```python
from build123d import *

# Parameters (mm, degrees)
SKETCH1_R           = 2.5
BOSS_EXTRUDE1_DEPTH = 2.5
BOSS_EXTRUDE2_START = -45
SKETCH4_R           = 3.5
SKETCH4_R_2         = 2
BOSS_EXTRUDE2_DEPTH = 47.5
BOSS_EXTRUDE3_START = -2.5
SKETCH5_R           = 2.5
BOSS_EXTRUDE3_DEPTH = 2.5
BOSS_EXTRUDE4_START = -12
BOSS_EXTRUDE4_DEPTH = 12
BOSS_EXTRUDE5_DEPTH = 2.5
FILLET2_R           = 1
FILLET3_R           = 1


with BuildPart() as part:
    # Sketch1 → Boss-Extrude1 (new body)
    with BuildSketch(Plane(origin=(0, 0, 0), x_dir=(1, 0, 0), z_dir=(0, 1, 0))):
        with BuildLine():
            Line((20.5, 10.5), (-20.5, 10.5))
            Line((-20.5, 10.5), (-20.5, 4))
            ThreePointArc((-20.5, 4), (-24.40287122, 1.76806345), (-28.520566145, 3.573204173))
            ThreePointArc((-28.520566145, 3.573204173), (-29.324072849, 5.171652721), (-29.350396575, 6.960498116))
            ThreePointArc((-29.350396575, 6.960498116), (-26.904940816, 10.941842627), (-22.5, 12.5))
            Line((-22.5, 12.5), (22.5, 12.5))
            ThreePointArc((22.5, 12.5), (26.904940816, 10.941842627), (29.350396575, 6.960498116))
            ThreePointArc((29.350396575, 6.960498116), (29.324072849, 5.171652721), (28.520566145, 3.573204173))
            ThreePointArc((28.520566145, 3.573204173), (25.737402548, 1.876578025), (22.5, 2.2557411))
            Line((22.5, 2.2557411), (22.5, -2.2557411))
            ThreePointArc((22.5, -2.2557411), (25.737402548, -1.876578025), (28.520566145, -3.573204173))
            ThreePointArc((28.520566145, -3.573204173), (29.324072849, -5.171652721), (29.350396575, -6.960498116))
            ThreePointArc((29.350396575, -6.960498116), (26.904940816, -10.941842627), (22.5, -12.5))
            Line((22.5, -12.5), (-22.5, -12.5))
            ThreePointArc((-22.5, -12.5), (-26.904940816, -10.941842627), (-29.350396575, -6.960498116))
            ThreePointArc((-29.350396575, -6.960498116), (-29.324072849, -5.171652721), (-28.520566145, -3.573204173))
            ThreePointArc((-28.520566145, -3.573204173), (-24.40287122, -1.76806345), (-20.5, -4))
            Line((-20.5, -4), (-20.5, -10.5))
            Line((-20.5, -10.5), (20.5, -10.5))
            Line((20.5, -10.5), (20.5, 10.5))
        make_face()
        with Locations(Location((-25, 5.5, 0), (0, 0, 270))):
            Circle(SKETCH1_R, mode=Mode.SUBTRACT)
        with Locations(Location((-25, -5.5, 0), (0, 0, 270))):
            Circle(SKETCH1_R, mode=Mode.SUBTRACT)
        with Locations(Location((25, -5.5, 0), (0, 0, 90))):
            Circle(SKETCH1_R, mode=Mode.SUBTRACT)
        with Locations(Location((25, 5.5, 0), (0, 0, 90))):
            Circle(SKETCH1_R, mode=Mode.SUBTRACT)
    extrude(amount=BOSS_EXTRUDE1_DEPTH)

    # Sketch4 → Boss-Extrude2 (add)
    # profile 1 of 4: a face of its own
    with BuildSketch(Plane(origin=(0, 0, 0), x_dir=(1, 0, 0), z_dir=(0, 1, 0)).offset(BOSS_EXTRUDE2_START)):
        with Locations(Location((-20.5, 15.5, 0), (0, 0, 270))):
            Circle(SKETCH4_R)
        with Locations(Location((-20.5, 15.5, 0), (0, 0, 270))):
            Circle(SKETCH4_R_2, mode=Mode.SUBTRACT)
    # profile 2 of 4: a face of its own
    with BuildSketch(Plane(origin=(0, 0, 0), x_dir=(1, 0, 0), z_dir=(0, 1, 0)).offset(BOSS_EXTRUDE2_START)):
        with Locations(Location((20.5, 15.5, 0), (0, 0, 270))):
            Circle(SKETCH4_R)
        with Locations(Location((20.5, 15.5, 0), (0, 0, 270))):
            Circle(SKETCH4_R_2, mode=Mode.SUBTRACT)
    # profile 3 of 4: a face of its own
    with BuildSketch(Plane(origin=(0, 0, 0), x_dir=(1, 0, 0), z_dir=(0, 1, 0)).offset(BOSS_EXTRUDE2_START)):
        with Locations(Location((-20.5, -15.5, 0), (0, 0, 270))):
            Circle(SKETCH4_R)
        with Locations(Location((-20.5, -15.5, 0), (0, 0, 270))):
            Circle(SKETCH4_R_2, mode=Mode.SUBTRACT)
    # profile 4 of 4: a face of its own
    with BuildSketch(Plane(origin=(0, 0, 0), x_dir=(1, 0, 0), z_dir=(0, 1, 0)).offset(BOSS_EXTRUDE2_START)):
        with Locations(Location((20.5, -15.5, 0), (0, 0, 270))):
            Circle(SKETCH4_R)
        with Locations(Location((20.5, -15.5, 0), (0, 0, 270))):
            Circle(SKETCH4_R_2, mode=Mode.SUBTRACT)
    extrude(amount=BOSS_EXTRUDE2_DEPTH)

    # Sketch5 → Boss-Extrude3 (add)
    with BuildSketch(Plane(origin=(0, 0, 0), x_dir=(1, 0, 0), z_dir=(0, 1, 0)).offset(BOSS_EXTRUDE3_START)):
        with BuildLine():
            Line((-29.324072849, 5.171652721), (-29.324072849, -5.171652721))
            ThreePointArc((-29.324072849, -5.171652721), (-29.438527194, -6.064584851), (-29.350396575, -6.960498116))
            ThreePointArc((-29.350396575, -6.960498116), (-27.465923203, -10.435821373), (-24, -12.337527971))
            Line((-24, -12.337527971), (-24, -15.5))
            Line((-24, -15.5), (-22.5, -15.5))
            ThreePointArc((-22.5, -15.5), (-20.5, -13.5), (-18.5, -15.5))
            Line((-18.5, -15.5), (-17, -15.5))
            Line((-17, -15.5), (-17, -12.5))
            Line((-17, -12.5), (17, -12.5))
            Line((17, -12.5), (17, -15.5))
            Line((17, -15.5), (18.5, -15.5))
            ThreePointArc((18.5, -15.5), (20.5, -13.5), (22.5, -15.5))
            Line((22.5, -15.5), (24, -15.5))
            Line((24, -15.5), (24, -12.337527971))
            ThreePointArc((24, -12.337527971), (27.465923203, -10.435821373), (29.350396575, -6.960498116))
            ThreePointArc((29.350396575, -6.960498116), (29.324072849, -5.171652721), (28.520566145, -3.573204173))
            ThreePointArc((28.520566145, -3.573204173), (25.737402548, -1.876578025), (22.5, -2.2557411))
            Line((22.5, -2.2557411), (22.5, 2.2557411))
            ThreePointArc((22.5, 2.2557411), (25.737402548, 1.876578025), (28.520566145, 3.573204173))
            ThreePointArc((28.520566145, 3.573204173), (29.324072849, 5.171652721), (29.350396575, 6.960498116))
            ThreePointArc((29.350396575, 6.960498116), (27.465923203, 10.435821373), (24, 12.337527971))
            Line((24, 12.337527971), (24, 15.5))
            Line((24, 15.5), (22.5, 15.5))
            ThreePointArc((22.5, 15.5), (20.5, 13.5), (18.5, 15.5))
            Line((18.5, 15.5), (17, 15.5))
            Line((17, 15.5), (17, 12.5))
            Line((17, 12.5), (-17, 12.5))
            Line((-17, 12.5), (-17, 15.5))
            Line((-17, 15.5), (-18.5, 15.5))
            ThreePointArc((-18.5, 15.5), (-20.5, 13.5), (-22.5, 15.5))
            Line((-22.5, 15.5), (-24, 15.5))
            Line((-24, 15.5), (-24, 12.337527971))
            ThreePointArc((-24, 12.337527971), (-27.465923203, 10.435821373), (-29.350396575, 6.960498116))
            ThreePointArc((-29.350396575, 6.960498116), (-29.438527194, 6.064584851), (-29.324072849, 5.171652721))
        make_face()
        with Locations(Location((-25, 5.5, 0), (0, 0, 270))):
            Circle(SKETCH5_R, mode=Mode.SUBTRACT)
        with Locations(Location((-25, -5.5, 0), (0, 0, 270))):
            Circle(SKETCH5_R, mode=Mode.SUBTRACT)
        with Locations(Location((25, -5.5, 0), (0, 0, 90))):
            Circle(SKETCH5_R, mode=Mode.SUBTRACT)
        with Locations(Location((25, 5.5, 0), (0, 0, 90))):
            Circle(SKETCH5_R, mode=Mode.SUBTRACT)
        with BuildLine():
            Line((-26.208643878, 2.004095257), (-26.208643878, -2.004095257))
            ThreePointArc((-26.208643878, -2.004095257), (-23.018368657, -2.041161266), (-20.5, -4))
            Line((-20.5, -4), (-20.5, -10.5))
            Line((-20.5, -10.5), (20.5, -10.5))
            Line((20.5, -10.5), (20.5, 10.5))
            Line((20.5, 10.5), (-20.5, 10.5))
            Line((-20.5, 10.5), (-20.5, 4))
            ThreePointArc((-20.5, 4), (-23.018368657, 2.041161266), (-26.208643878, 2.004095257))
        make_face(mode=Mode.SUBTRACT)
    extrude(amount=BOSS_EXTRUDE3_DEPTH)

    # Sketch6 → Boss-Extrude4 (add)
    with BuildSketch(Plane(origin=(0, 0, 0), x_dir=(1, 0, 0), z_dir=(0, 1, 0)).offset(BOSS_EXTRUDE4_START)):
        with BuildLine():
            Line((-24, 15.5), (-22.5, 15.5))
            ThreePointArc((-22.5, 15.5), (-20.5, 13.5), (-18.5, 15.5))
            Line((-18.5, 15.5), (-17, 15.5))
            Line((-17, 15.5), (-17, 12.5))
            Line((-17, 12.5), (17, 12.5))
            Line((17, 12.5), (17, 15.5))
            Line((17, 15.5), (18.5, 15.5))
            ThreePointArc((18.5, 15.5), (20.5, 13.5), (22.5, 15.5))
            Line((22.5, 15.5), (24, 15.5))
            Line((24, 15.5), (24, 10.1))
            Line((24, 10.1), (-24, 10.1))
            Line((-24, 10.1), (-24, 15.5))
        make_face()
        with BuildLine():
            Line((24, -15.5), (24, -10.1))
            Line((24, -10.1), (-24, -10.1))
            Line((-24, -10.1), (-24, -15.5))
            Line((-24, -15.5), (-22.5, -15.5))
            ThreePointArc((-22.5, -15.5), (-20.5, -13.5), (-18.5, -15.5))
            Line((-18.5, -15.5), (-17, -15.5))
            Line((-17, -15.5), (-17, -12.5))
            Line((-17, -12.5), (17, -12.5))
            Line((17, -12.5), (17, -15.5))
            Line((17, -15.5), (18.5, -15.5))
            ThreePointArc((18.5, -15.5), (20.5, -13.5), (22.5, -15.5))
            Line((22.5, -15.5), (24, -15.5))
        make_face()
    extrude(amount=BOSS_EXTRUDE4_DEPTH)

    # Sketch7 → Boss-Extrude5 (add)
    with BuildSketch(Plane(origin=(0, 0, 0), x_dir=(1, 0, 0), z_dir=(0, 1, 0))):
        with BuildLine():
            Line((-24, -15.5), (-24, -10.98088563))
            Line((-24, -10.98088563), (-17, -10.98088563))
            Line((-17, -10.98088563), (-17, -15.5))
            ThreePointArc((-17, -15.5), (-20.5, -12), (-24, -15.5))
        make_face()
        with BuildLine():
            Line((17, -15.5), (17, -10.98088563))
            Line((17, -10.98088563), (24, -10.98088563))
            Line((24, -10.98088563), (24, -15.5))
            ThreePointArc((24, -15.5), (20.5, -12), (17, -15.5))
        make_face()
        with BuildLine():
            Line((24, 10.98088563), (24, 15.5))
            ThreePointArc((24, 15.5), (20.5, 12), (17, 15.5))
            Line((17, 15.5), (17, 10.98088563))
            Line((17, 10.98088563), (24, 10.98088563))
        make_face()
        with BuildLine():
            Line((-24, 10.98088563), (-17, 10.98088563))
            Line((-17, 10.98088563), (-17, 15.5))
            ThreePointArc((-17, 15.5), (-20.5, 12), (-24, 15.5))
            Line((-24, 15.5), (-24, 10.98088563))
        make_face()
    extrude(amount=BOSS_EXTRUDE5_DEPTH)

    # Fillet2
    # the kernel refuses this fillet: 1 mm, written as the material it adds along each edge
    with BuildSketch(Plane(origin=(-22.5, 0, -10.5), x_dir=(0, 1, 0), z_dir=(1, 0, 0))) as fillet2_piece_1:
        with BuildLine():
            CenterArc((0.8, 1), FILLET2_R, 216.869897646, 53.130102354)
            Line((0, 0.4), (-0.016, 0.388))
            ThreePointArc((-0.016, 0.388), (-0.02, 0.2), (-0.02, 0))
            Line((-0.02, 0), (0, -0.02))
            Line((0, -0.02), (0.8, -0.02))
            Line((0.8, -0.02), (0.8, 0))
        make_face()
    extrude(amount=45)

    # Fillet3
    # the kernel refuses this fillet: 1 mm, written as the material it adds along each edge
    with BuildSketch(Plane(origin=(-22.5, 0, 10.5), x_dir=(0, 0, -1), z_dir=(1, 0, 0))) as fillet3_piece_1:
        with BuildLine():
            CenterArc((1, 0.8), FILLET3_R, 180, 53.130102354)
            Line((0, 0.8), (-0.02, 0.8))
            Line((-0.02, 0.8), (-0.02, 0))
            Line((-0.02, 0), (0, -0.02))
            ThreePointArc((0, -0.02), (0.2, -0.02), (0.388, -0.016))
            Line((0.388, -0.016), (0.4, 0))
        make_face()
    extrude(amount=45)


solid = part.part
```
For this review, take the finished solid that the model builds, in its own axes (mm). A direction names the side the tool comes from. Round coordinates to 2 decimals unless told otherwise and drop trailing zeros. Write each loop counter-clockwise with the first axis right and the second up, starting at its lowest first coordinate (ties: lowest second). Pieces come first, ordered by that corner, then holes. Notation, with made-up numbers: (78, 10.5) - (83, 10.5) arc R21 cw to (83, 49.5) - close; hole circle Ø3 at (84, 9.5). An arc over 180 degrees is marked (long way). Write each question's results on one line, items separated by ' | '.
Item 1: Take a section at C-C on x = 7. State the section outline as (y, z) points, then the cut area to 3 significant figures.
Calculated:
outline: (-12, -12.5) - (2.5, -12.5) - (2.5, -10.5) - (0.8, -10.5) arc R1 cw to (0, -10.1) - (-12, -10.1) - close; (-12, 10.1) - (0, 10.1) arc R1 cw to (0.8, 10.5) - (2.5, 10.5) - (2.5, 12.5) - (-12, 12.5) - close | area: 67.8 mm^2
Item 2: Take a section at A-A on y = -21. State the section outline as (x, z) points, then the cut area to 3 significant figures.
Calculated:
outline: circle Ø7 at (-20.5, -15.5); circle Ø7 at (-20.5, 15.5); circle Ø7 at (20.5, -15.5); circle Ø7 at (20.5, 15.5); hole circle Ø4 at (-20.5, -15.5); hole circle Ø4 at (-20.5, 15.5); hole circle Ø4 at (20.5, -15.5); hole circle Ø4 at (20.5, 15.5) | area: 104 mm^2
Item 3: For pin 1 (8 mm diameter, centred on y = -14, z = -11, fed in from -X); pin 2 (10 mm diameter, centred on x = 27, z = -2.5, fed in from -Y); pin 3 (0.5 mm diameter, centred on x = -5, y = 1.5, fed in from -Z); pin 4 (12 mm diameter, centred on y = -30.5, z = 4, fed in from -X), all flat-tipped, find the tip position at first contact; note any pin that passes through.
Calculated:
pin 1: stops at x = -24 | pin 2: stops at y = -2.5 | pin 3: stops at z = -12.5 | pin 4: passes through
Item 4: Draft analysis for pull direction X (two halves, no side actions). For faces 1 (the face through (-24, -6, -13)), 2 (the face through (0, 2, 10.5)), 3 (the face through (29.33, -0.04, 5.2)), state which applies: pulls with the +X half, pulls with the -X half, needs draft (parallel to the pull), parting line crosses it, or undercut.
Calculated:
face 1: pulls with the -X half | face 2: undercut | face 3: pulls with the +X half
Item 5: For faces 4 (the face through (-29.324, -1, 0)), 5 (the face through (0, -5, -12.5)), 6 (the face through (24, -6, 13)), list the 3-axis set-ups (+Z, -Z, +X, -X, +Y, -Y) from which the entire face can be reached by the end or side of a thin tool; tool diameter is ignored.
Calculated:
face 4: -X, +Y, -Y | face 5: -Z, +Y, -Y | face 6: +Z, +X, -Y
Item 6: Take a section at B-B on z = 16.5. State the section outline as (x, y) points, then the cut area to 3 significant figures.
Calculated:
outline: (-23.85, -45) - (-22.23, -45) - (-22.23, 2.5) - (-23.85, 2.5) - close; (-18.77, -45) - (-17.15, -45) - (-17.15, 2.5) - (-18.77, 2.5) - close; (17.15, -45) - (18.77, -45) - (18.77, 2.5) - (17.15, 2.5) - close; (22.23, -45) - (23.85, -45) - (23.85, 2.5) - (22.23, 2.5) - close | area: 308 mm^2
Item 7: Take a section at D-D on x = -25. State the section outline as (y, z) points.
Calculated:
outline: (-2.5, -12.04) - (2.5, -12.04) - (2.5, -8) - (-2.5, -8) - close; (-2.5, -3) - (2.5, -3) - (2.5, -1.77) - (-2.5, -1.77) - close; (-2.5, 1.77) - (2.5, 1.77) - (2.5, 3) - (-2.5, 3) - close; (-2.5, 8) - (2.5, 8) - (2.5, 12.04) - (-2.5, 12.04) - close
Item 8: To check wall thickness, follow line 1 along Z through (x, y) = (-0.5, -2.5); line 2 along Z through (x, y) = (25, 0.8); line 3 along X through (y, z) = (-31, -15). State the ranges of each line that lie inside material, in increasing order. Write a range as from..to.
Calculated:
line 1: z = -12.5..-10.1, 10.1..12.5 | line 2: z = -12.04..-8, -3..-1.77, 1.77..3, 8..12.04 | line 3: x = -23.96..-22.44, -18.56..-17.04, 17.04..18.56, 22.44..23.96
